Geometry: final body of the model. Coordinates: model frame, mm. Give positions to 0.01 mm unless a question says otherwise; leave off trailing zeros. Write each loop counter-clockwise with the first axis right and the second up, starting at its lowest first coordinate (ties: lowest second). Pieces come first, ordered by that corner, then holes. Notation, with made-up numbers: (-14.75, 55) -> (19.25, 55) arc R21 ccw to (19.25, 61) -> close; hole circle Ø7 at (-13, 5.5). An arc over 180 degrees is marked (long way). Answer in a Markdown table with one row per item. Add a question column.
Item 1: Section query B-B on y = 0. Output: boundary loops of the cut face in (x, z), plus the area to 3 significant figures.
Item 2: Section query A-A on z = 345. Output: boundary loops of the cut face in (x, y), plus the area to 3 significant figures.
Item 3: Section query D-D on z = 38. Output: boundary loops of the cut face in (x, y), plus the area to 3 significant figures.
Item 4: Section query C-C on z = -25.5. Output: boundary loops of the cut face in (x, y), plus the area to 3 significant figures.
Item 5: Material intervals for probe 1 along Z at (x, y) = (0, -10.5); probe 2 along Y at (x, z) = (5, 332.5); probe 3 along Z at (x, y) = (0, 1), sorted ascending. Write a range as from..to.
Item 6: First-contact query: P1, Ø16, axis at y = 21, z = 333, coming from the -X side; P2, Ø18.5, axis at y = -11, z = 341.5, coming from the -X side; P3, Ø11.5, axis at y = 2, z = -8, coming from the +X side. Flat tips, straight axial feed; report the tip coordinate or a pass-through.
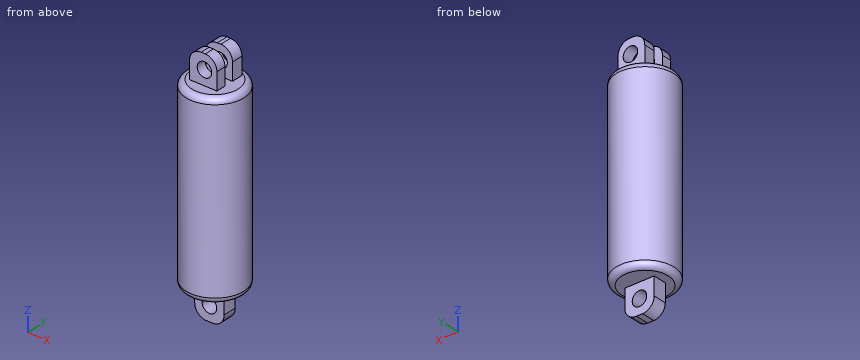
```python
from build123d import *

# Parameters (mm, degrees)
F0_R     = 50
F1_DEPTH = 320
F2_W     = 47.244698
F2_H     = 16.991875
F2_W_2   = 46.056544
F2_H_2   = 20.037373
F3_DEPTH = 50
F4_R     = 12.5
F5_DEPTH = 72.138193
F6_W     = 50.61818
F6_H     = 23.403664
F7_DEPTH = 51
F8_R     = 12.5
F9_DEPTH = 61.702832
F10_R    = 20
F11_R    = 10


with BuildPart() as f1:
    # F0 (on Top) → F1 (new body)
    with BuildSketch(Plane.XY):
        Circle(F0_R)
    extrude(amount=F1_DEPTH)

    # F2 (on face) → F3 (join)
    with BuildSketch(Plane.XY.offset(320)):
        with Locations((-2.225159, -13.641255)):
            Rectangle(F2_W, F2_H)
        with Locations((-1.631082, 20.769891)):
            Rectangle(F2_W_2, F2_H_2)
    extrude(amount=F3_DEPTH)

    # F4 (on face) → F5 (cut, through all)
    with BuildSketch(Plane.XZ.offset(22.137193)):
        with Locations((0, 345)):
            Circle(F4_R)
    extrude(amount=-F5_DEPTH, mode=Mode.SUBTRACT)

    # F6 (on Top) → F7 (join)
    with BuildSketch(Plane.XY):
        Rectangle(F6_W, F6_H)
    extrude(amount=-F7_DEPTH)

    # F8 (on face) → F9 (cut, through all)
    with BuildSketch(Plane(origin=(0, 11.701832, 0), x_dir=(-1, 0, 0), z_dir=(0, 1, 0))):
        with Locations((0, -25.5)):
            Circle(F8_R)
    extrude(amount=-F9_DEPTH, mode=Mode.SUBTRACT)

    # F10
    f10_edges = [f1.edges().sort_by_distance(p)[0] for p in [
        (21.39719, -13.641255, 370),
        (21.39719, 20.769892, 370),
        (-24.659354, 20.769892, 370),
        (-25.847508, -13.641255, 370),
        (25.30909, 0, -51),
        (-25.30909, 0, -51),
    ]]
    fillet(f10_edges, radius=F10_R)

    # F11
    f11_edges = [f1.edges().sort_by_distance(p)[0] for p in [
        (-50, 0, 0),
        (-50, 0, 320),
    ]]
    fillet(f11_edges, radius=F11_R)


solid = f1.part
```
Findings below:
| question | item | result |
|---|---|---|
| 1 | outline | (-50, 10) arc R10 ccw to (-40, 0) -> (-25.31, 0) -> (-25.31, -31) arc R20 ccw to (-5.31, -51) -> (5.31, -51) arc R20 ccw to (25.31, -31) -> (25.31, 0) -> (40, 0) arc R10 ccw to (50, 10) -> (50, 310) arc R10 ccw to (40, 320) -> (-40, 320) arc R10 ccw to (-50, 310) -> close; hole circle Ø25 at (0, -25.5) |
| 1 | area | 33,800 mm^2 |
| 2 | outline | (-25.85, -22.14) -> (-12.5, -22.14) -> (-12.5, -5.15) -> (-25.85, -5.15) -> close; (-24.66, 10.75) -> (-12.5, 10.75) -> (-12.5, 30.79) -> (-24.66, 30.79) -> close; (12.5, -22.14) -> (21.4, -22.14) -> (21.4, -5.15) -> (12.5, -5.15) -> close; (12.5, 10.75) -> (21.4, 10.75) -> (21.4, 30.79) -> (12.5, 30.79) -> close |
| 2 | area | 800 mm^2 |
| 3 | outline | circle Ø100 at (0, 0) |
| 3 | area | 7,850 mm^2 |
| 4 | outline | (-25.31, -11.7) -> (-12.5, -11.7) -> (-12.5, 11.7) -> (-25.31, 11.7) -> close; (12.5, -11.7) -> (25.31, -11.7) -> (25.31, 11.7) -> (12.5, 11.7) -> close |
| 4 | area | 600 mm^2 |
| 5 | probe 1 | z = -51..-38, -13..332.5, 357.5..370 |
| 5 | probe 2 | y = -22.14..-5.15, 10.75..30.79 |
| 5 | probe 3 | z = -51..-38, -13..320 |
| 6 | P1 | stops at x = -24.66 |
| 6 | P2 | stops at x = -25.85 |
| 6 | P3 | stops at x = 25.31 |
